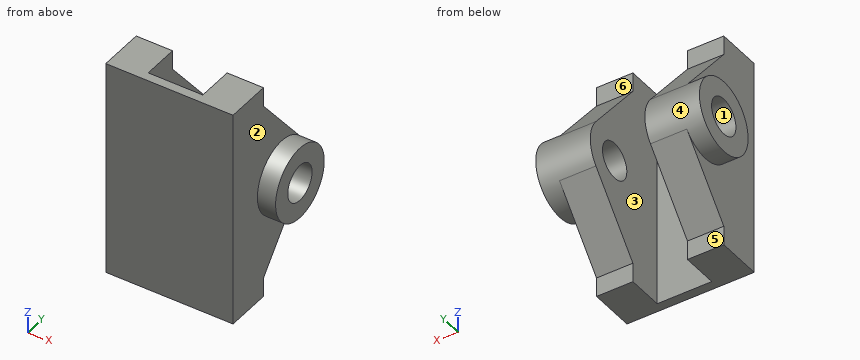
```python
from build123d import *

# Parameters (mm, degrees)
SKETCH1_W           = 70
SKETCH1_H           = 120
BOSS_EXTRUDE1_DEPTH = 25
SKETCH2_W           = 30
SKETCH2_H           = 120
CUT_EXTRUDE1_DEPTH  = 20
SKETCH4_R           = 20
SKETCH4_R_2         = 10
BOSS_EXTRUDE2_DEPTH = 30
BOSS_EXTRUDE3_DEPTH = 20


with BuildPart() as part:
    # Sketch1 → Boss-Extrude1 (new body)
    with BuildSketch(Plane(origin=(0, 0, 0), x_dir=(1, 0, 0), z_dir=(0, 1, 0))):
        Rectangle(SKETCH1_W, SKETCH1_H)
    extrude(amount=BOSS_EXTRUDE1_DEPTH)

    # Sketch2 → Cut-Extrude1 (cut)
    with BuildSketch(Plane(origin=(0, 25, 0), x_dir=(1, 0, 0), z_dir=(0, 1, 0))):
        Rectangle(SKETCH2_W, SKETCH2_H)
    extrude(amount=-CUT_EXTRUDE1_DEPTH, mode=Mode.SUBTRACT)

    # Sketch4 → Boss-Extrude2 (add)
    with BuildSketch(Plane(origin=(45, 0, 0), x_dir=(0, 0, -1), z_dir=(1, 0, 0))):
        with Locations((0, 40)):
            Circle(SKETCH4_R)
        with Locations((0, 40)):
            Circle(SKETCH4_R_2, mode=Mode.SUBTRACT)
    boss_extrude2 = extrude(amount=-BOSS_EXTRUDE2_DEPTH)

    # Mirror1: Boss-Extrude2 across plane
    add(boss_extrude2.mirror(Plane(origin=(0, 0, 0), x_dir=(0, 0, 1), z_dir=(1, 0, 0))))

    # Sketch5 → Boss-Extrude3 (add)
    with BuildSketch(Plane.ZY.offset(35)):
        with BuildLine():
            ThreePointArc((-13.228756555, 25), (-19.997722926, 40.301790929), (-12.770097474, 55.392355587))
            Line((-12.770097474, 55.392355587), (-49.403329543, 25))
            Line((-49.403329543, 25), (-13.228756555, 25))
        make_face()
        with BuildLine():
            Line((49.403329543, 25), (12.770097474, 55.392355587))
            ThreePointArc((12.770097474, 55.392355587), (18.10251294, 48.50288335), (20, 40))
            ThreePointArc((20, 40), (18.228756555, 31.771243445), (13.228756555, 25))
            Line((13.228756555, 25), (49.403329543, 25))
        make_face()
    boss_extrude3 = extrude(amount=-BOSS_EXTRUDE3_DEPTH)

    # Mirror2: Boss-Extrude3 across plane
    add(boss_extrude3.mirror(Plane(origin=(0, 0, 0), x_dir=(0, 0, 1), z_dir=(1, 0, 0))))


solid = part.part
```
Design review of the part built by this model. Coordinates are the model's own, in mm. Face numbers are marked on the shaded views. A direction names the side the tool comes from. Give positions to 0.01 mm unless a question says otherwise; leave off trailing zeros. Loops run counter-clockwise (first coordinate to the right, second up) from the corner with the lowest first, then second, coordinate; pieces in that order, holes last. Notation, with made-up numbers: M 65,49 L 86,49 A21 ccw 86,67 Z; hole C 69.5,30.25 d10. An arc over 180 degrees is marked long. Return JSON: item names as keys, results as strings. Group by question number.
Item 1: We need section B-B (y = 14). Give the boundary of the cut face in (x, z), and give its area (3 significant figures).
Item 2: We need section D-D (x = -3). Give the boundary of the cut face in (y, z).
Item 3: For probe 1 along Y at (x, z) = (-37.75, 0); probe 2 along X at (y, z) = (35, -34); probe 3 along X at (y, z) = (24.5, 8.5), list the stretches that pass through material, from the lowest coordinate up.
Item 4: Mouldability with a two-part tool opening along X and no side actions: class the marked faces 1, 2 and 3 as released by +X, released by -X, zero draft, split by the parting line, or undercut.
Item 5: We need section A-A (z = 0). Give the boundary of the cut face in (x, y).
Item 6: Tool access review of the marked faces 4, 5 and 6: name each direction out of +Z, -Z, +X, -X, +Y, -Y from which nothing blocks a thin tool from reaching the whole face with its end or side.
Item 7: Insertion check: pin 1 Ø2 at (y, z) = (43.5, -24) entering from -X; pin 2 Ø8.5 at (x, z) = (24, -55) entering from +Y; pin 3 Ø8.5 at (x, z) = (23, 52.5) entering from +Y. Each pin has a flat end and moves straight along its axis. Give the tip position at first contact, or say it passes through.
Item 8: We need section C-C (y = 40). Give the boundary of the cut face in (x, z), and give its area (3 significant figures).
Output:
{
 "1": {"outline": "M -35,-60 L -15,-60 L -15,60 L -35,60 Z; M 15,-60 L 35,-60 L 35,60 L 15,60 Z", "area": "4,800 mm^2"},
 "2": {"outline": "M 0,-60 L 5,-60 L 5,60 L 0,60 Z"},
 "3": {"probe 1": "y = 20 to 30, 50 to 60", "probe 2": "x = -35 to -15, 15 to 35", "probe 3": "x = -45 to -15, 15 to 45"},
 "4": {"face 1": "zero draft", "face 2": "released by +X", "face 3": "undercut"},
 "5": {"outline": "M -45,20 L -35,20 L -35,0 L 35,0 L 35,20 L 45,20 L 45,30 L 15,30 L 15,5 L -15,5 L -15,30 L -45,30 Z; M -45,50 L -15,50 L -15,60 L -45,60 Z; M 15,50 L 45,50 L 45,60 L 15,60 Z"},
 "6": {"face 4": "-X", "face 5": "-Z, +X, -X, +Y", "face 6": "+Z, +X, -X, +Y"},
 "7": {"pin 1": "stops at x = -35", "pin 2": "stops at y = 25", "pin 3": "stops at y = 25.96"},
 "8": {"outline": "M -45,-20 L -35,-20 L -35,-31.32 L -15,-31.32 L -15,-10 L -45,-10 Z; M -45,10 L -15,10 L -15,31.32 L -35,31.32 L -35,20 L -45,20 Z; M 15,-31.32 L 35,-31.32 L 35,-20 L 45,-20 L 45,-10 L 15,-10 Z; M 15,10 L 45,10 L 45,20 L 35,20 L 35,31.32 L 15,31.32 Z", "area": "2,110 mm^2"}
}
